Geometry check sheet. Reference: the model listing, model coordinates, mm. Coordinates: 2 decimals unless noted, no trailing zeros. Order: outer loops, then holes, each group sorted by start corner. A loop starts at its lowest first (then second) coordinate and runs counter-clockwise, first axis right, second up. Notation, with made-up numbers: M 67,39 L 120,39 A19 ccw 120,75 Z; hole C 66,10 d7. An arc over 180 degrees is marked long. One line per item, written item: value. Start each with the question number.
1) Draft check along Z on faces 1 (the cylindrical face through (-18.33, 0.49, -44.26)), 2 (the flat face through (-32, 0, -35)), 3 (the cylindrical face through (-20.117, 0.507, -54.815)). Enter one of: pulls with the +Z half, pulls with the -Z half, needs draft (parallel to the pull), parting line crosses it, or undercut.
2) Thickness scan on L1, parallel to Z at x = -32.75, y = 0.3; L2, parallel to Z at x = -19.5, y = 0.8; L3, parallel to X at y = 0.25, z = -42.59. Record the ranges inside material, lowest first. Write a range as from..to.
3) Sectioned sample at D-D, the plane z = -49. Enter the section's corners in (x, y), then the cut area to 3 significant figures.
4) Sectioned sample at B-B, the plane y = 0.5. Enter the section's corners in (x, z), then the cut area to 3 significant figures.
5) Go/stop test with a flat-tipped pin: P1, Ø2.5, axis at x = -19.6, z = -42.59, coming from the +Y side. Record where the tip stops, or that it passes through.
6) Sectioned sample at A-A, the plane x = -32.75. Enter the section's corners in (y, z).
7) Sectioned sample at C-C, the plane z = -26. Enter the section's corners in (x, y).
Autodesk Inventor part; units mm, degrees
ref_plane "YZ Plane" through (0, 0, 0) normal (1, 0, 0) x (0, 1, 0)
ref_plane "XZ Plane" through (0, 0, 0) normal (0, 1, 0) x (-1, 0, 0)
ref_plane "XY Plane" through (0, 0, 0) normal (0, 0, 1) x (1, 0, 0)
sketch "スケッチ1" plane through (0, 0, 0) normal (0, 1, 0) x (-1, 0, 0)
  line L0 (0, 0) -> (65.5, 0)
  line L1 (65.5, 0) -> (65.5, -70)
  line L2 (65.5, -70) -> (0, -70)
  line L3 (0, -70) -> (0, 0)
  dimension "d0" = 65.5
  dimension "d1" = 70
extrude "押し出し1" add sketch "スケッチ1" along normal blind 1
sketch "スケッチ3" plane through (0, 1, 0) normal (0, 1, 0) x (1, 0, 0)
  line L0 (-65.5, 0) -> (0, 0)
  line L1 (-32.75, 0) -> (-32.75, 70)
  line L2 (0, 70) -> (-65.5, 70)
  circle A0 centre (-32.75, 35) radius 15.18
  point P0 (-32.75, 50.18)
  point P1 (-45.8963, 42.59)
  point P2 (-45.8963, 27.41)
  point P3 (-32.75, 19.82)
  point P4 (-19.6037, 27.41)
  point P5 (-19.6037, 42.59)
  dimension "d15" = 30.36
  dimension "d18" = 360
hole "穴2" at (-32.75, 1, -50.18) at (-45.8963, 1, -42.59) at (-45.8963, 1, -27.41) at (-32.75, 1, -19.82) at (-19.6037, 1, -27.41) at (-19.6037, 1, -42.59) direction (0, -1, 0) diameter 4.2 end through all
sketch "スケッチ4" plane through (0, 1, 0) normal (0, 1, 0) x (1, 0, 0)
  line L0 (-65.5, 70) -> (-65.5, 0)
  line L1 (0, 70) -> (-65.5, 70)
  circle A0 centre (-32.75, 35) radius 23.5
  line L2 (0, 0) -> (0, 70)
  line L3 (-65.5, 70) -> (0, 70)
  line L4 (0, 70) -> (0, 0)
  line L5 (0, 0) -> (-65.5, 0)
  line L6 (-65.5, 0) -> (-65.5, 70)
  dimension "d27" = 47
  dimension "d28" = 35
  dimension "d29" = 32.75
extrude "押し出し2" cut sketch "スケッチ4" against normal blind 1
properties part number "link2_plate5" material "アルミニウム 6061"
Final values:
1. face 1: undercut
1. face 2: needs draft
1. face 3: parting line crosses it
2. L1: z = -58.5..-52.28, -48.08..-21.92, -17.72..-11.5
2. L2: z = -54.41..-44.69, -40.49..-29.51, -25.31..-15.59
2. L3: x = -54.99..-48, -43.8..-21.7, -17.5..-10.51
3. outline: M -51.62,0 L -34.49,0 L -34.49,1 L -51.62,1 Z; M -31.01,0 L -13.88,0 L -13.88,1 L -31.01,1 Z
3. area: 34.3 mm^2
4. outline: C -32.75,-35 d47; hole C -45.9,-42.59 d4.2; hole C -45.9,-27.41 d4.2; hole C -32.75,-50.18 d4.2; hole C -32.75,-19.82 d4.2; hole C -19.6,-42.59 d4.2; hole C -19.6,-27.41 d4.2
4. area: 1,650 mm^2
5. P1: passes through
6. outline: M 0,-58.5 L 1,-58.5 L 1,-52.28 L 0,-52.28 Z; M 0,-48.08 L 1,-48.08 L 1,-21.92 L 0,-21.92 Z; M 0,-17.72 L 1,-17.72 L 1,-11.5 L 0,-11.5 Z
7. outline: M -54.46,0 L -47.45,0 L -47.45,1 L -54.46,1 Z; M -44.34,0 L -21.16,0 L -21.16,1 L -44.34,1 Z; M -18.05,0 L -11.04,0 L -11.04,1 L -18.05,1 Z
